Can you work these out from the model? Positions are in its coordinate system, mm. Round coordinates to 2 decimals unless told otherwise and drop trailing zeros. Loops run counter-clockwise (first coordinate to the right, second up) from the corner with the lowest first, then second, coordinate; pieces in that order, holes last. Notation, with made-up numbers: (-16, 38) -> (7, 38) arc R31 cw to (7, 62) -> close; hole circle Ø10 at (40, 17). An arc over 180 degrees is marked (long way). Answer as a JSON object with one key per item and string values.
```python
from build123d import *

# Parameters (mm, degrees)
SKETCH1_R           = 40
BOSS_EXTRUDE1_DEPTH = 209.644706
SKETCH2_R           = 23.059697106
CUT_EXTRUDE1_DEPTH  = 218.142586228
CHAMFER1_SIZE       = 2.680415


with BuildPart() as part:
    # Sketch1 → Boss-Extrude1 (new body)
    with BuildSketch(Plane(origin=(0, 0, 0), x_dir=(1, 0, 0), z_dir=(0, 1, 0))):
        with Locations(Location((0, 0, 0), (0, 0, 270))):
            Circle(SKETCH1_R)
    extrude(amount=BOSS_EXTRUDE1_DEPTH)

    # Sketch2 → Cut-Extrude1 (cut, through all)
    with BuildSketch(Plane(origin=(0, 0, 0), x_dir=(1, 0, 0), z_dir=(0, 1, 0))):
        with Locations(Location((0, 0, 0), (0, 0, 270))):
            Circle(SKETCH2_R)
    extrude(amount=CUT_EXTRUDE1_DEPTH, mode=Mode.SUBTRACT)

    # Chamfer1
    chamfer1_edges = [part.edges().sort_by_distance(p)[0] for p in [
        (0, 0, -40),
        (0, 209.644706, -40),
        (0, 0, -23.059697106),
        (0, 209.644706, -23.059697106),
    ]]
    chamfer(chamfer1_edges, length=CHAMFER1_SIZE)


solid = part.part
```
Q1. I want a section at B-B, the plane x = 0. Write out the boundary of the cut face in (y, z).
Determined:
{"outline": "(0, -37.32) -> (2.68, -40) -> (206.96, -40) -> (209.64, -37.32) -> (209.64, -25.74) -> (206.96, -23.06) -> (2.68, -23.06) -> (0, -25.74) -> close; (0, 25.74) -> (2.68, 23.06) -> (206.96, 23.06) -> (209.64, 25.74) -> (209.64, 37.32) -> (206.96, 40) -> (2.68, 40) -> (0, 37.32) -> close"}
Q2. I want a section at A-A, the plane z = 0. Write out the boundary of the cut face in (x, y).
Determined:
{"outline": "(-40, 2.68) -> (-37.32, 0) -> (-25.74, 0) -> (-23.06, 2.68) -> (-23.06, 206.96) -> (-25.74, 209.64) -> (-37.32, 209.64) -> (-40, 206.96) -> close; (23.06, 2.68) -> (25.74, 0) -> (37.32, 0) -> (40, 2.68) -> (40, 206.96) -> (37.32, 209.64) -> (25.74, 209.64) -> (23.06, 206.96) -> close"}
Q3. I'm going to push flat-ended pins straight in: pin 1 (1 mm diameter, centred on x = -29.5, y = 28.5, fed in from -Z); pin 2 (4 mm diameter, centred on x = -16.5, y = 136.5, fed in from +Z); pin 3 (10 mm diameter, centred on x = -8, y = 61.5, fed in from -Z). Where does each tip first touch, or does it pass through?
Determined:
{"pin 1": "z = -27.55", "pin 2": "z = 37.28", "pin 3": "z = -39.89"}
Q4. If I drill on L1, parallel to X at y = 129.5, z = 0; L2, parallel to X at y = 74, z = 5.5; L3, parallel to Z at x = 13, y = 55.5, over which ranges is the centre line in solid material (lowest first)? Write a range as [from, to].
Determined:
{"L1": "[-40, -23.06], [23.06, 40]", "L2": "[-39.62, -22.39], [22.39, 39.62]", "L3": "[-37.83, -19.05], [19.05, 37.83]"}
Q5. We'd pull the mould along X, two halves only. Please class faces 1 (the conical face through (22.638, 207.094, -5.027)), 2 (the cylindrical face through (-39.05, 103.39, -8.67)), 3 (the flat face through (-24.4, 209.645, -8.8)): pulls with the +X half, pulls with the -X half, needs draft (parallel to the pull), parting line crosses it, or undercut.
Determined:
{"face 1": "undercut", "face 2": "parting line crosses it", "face 3": "needs draft"}
Q6. I want a section at C-C, the plane y = 175. Write out the boundary of the cut face in (x, z), then the cut area to 3 significant figures.
Determined:
{"outline": "circle Ø80 at (0, 0); hole circle Ø46.12 at (0, 0)", "area": "3,360 mm²"}
